from build123d import *

# Parameters (mm, degrees)
CROQUIS2_W              = 50
CROQUIS2_H              = 50
SALIENTE_EXTRUIR1_DEPTH = 1.4
CROQUIS3_R              = 1.6
CORTAR_EXTRUIR1_DEPTH   = 1.4
CROQUIS4_W              = 50
CROQUIS4_H              = 32.2
SALIENTE_EXTRUIR2_DEPTH = 23.2
SALIENTE_EXTRUIR3_DEPTH = 14.6
CROQUIS6_R              = 5
SALIENTE_EXTRUIR4_DEPTH = 16.4


with BuildPart() as part:
    # Croquis2 → Saliente-Extruir1 (new body)
    with BuildSketch(Plane.XY):
        Rectangle(CROQUIS2_W, CROQUIS2_H)
    extrude(amount=SALIENTE_EXTRUIR1_DEPTH)

    # Croquis3 → Cortar-Extruir1 (cut)
    with BuildSketch(Plane.XY.offset(1.4)):
        with Locations((20.4, 22)):
            Circle(CROQUIS3_R)
        with Locations((20.4, -18)):
            Circle(CROQUIS3_R)
        with Locations((-18.1, 22)):
            Circle(CROQUIS3_R)
        with Locations((-18.1, -18)):
            Circle(CROQUIS3_R)
    extrude(amount=-CORTAR_EXTRUIR1_DEPTH, mode=Mode.SUBTRACT)

    # Croquis4 → Saliente-Extruir2 (add)
    with BuildSketch(Plane(origin=(0, 0, 0), x_dir=(-1, 0, 0), z_dir=(0, 0, -1))):
        with Locations((0, 2.75)):
            Rectangle(CROQUIS4_W, CROQUIS4_H)
    extrude(amount=SALIENTE_EXTRUIR2_DEPTH)

    # Croquis5 → Saliente-Extruir3 (add)
    with BuildSketch(Plane.XY.offset(1.4)):
        Polygon((-14.1, -18), (-14.1, -25), (5.9, -25), (5.9, -15), (-14.1, -15), align=None)
    extrude(amount=SALIENTE_EXTRUIR3_DEPTH)

    # Croquis6 → Saliente-Extruir4 (add)
    with BuildSketch(Plane.XY.offset(1.4)):
        with Locations(Location((11.9, -20, 0), (0, 0, 270))):
            Circle(CROQUIS6_R)
    extrude(amount=SALIENTE_EXTRUIR4_DEPTH)


solid = part.part
Check sheet for the modelled part. Datum: model origin and axes. Units: mm. A direction names the side the tool comes from. Round coordinates to 2 decimals unless told otherwise and drop trailing zeros. Loops run counter-clockwise (first coordinate to the right, second up) from the corner with the lowest first, then second, coordinate; pieces in that order, holes last. Notation, with made-up numbers: M -30.75,38.25 L 25.25,38.25 A16 cw 25.25,48.25 Z; hole C 52.25,64 d10. An arc over 180 degrees is marked long. One line per question, with ' | ' between items. Start each with the question number.
Item 1: Section check D-D (x = -2). Record the boundary of the cut face in (y, z).
Item 2: Scan lines: probe 1 along Y at (x, z) = (20.4, 0.6); probe 2 along Y at (x, z) = (5.5, 7.5); probe 3 along Y at (x, z) = (-22, -12.5). Record each from-to range of solid material in increasing order.
Item 3: Section check C-C (z = 12). Record the boundary of the cut face in (x, y), and give its area (3 significant figures).
Item 4: Section check A-A (y = 22). Record the boundary of the cut face in (x, z).
Item 5: Section check B-B (x = -18.1). Record the boundary of the cut face in (y, z).
Item 6: Set-up check for faces 1 (the face through (-4, -20, 16)), 2 (the face through (-4, -15, 9)), 3 (the face through (0, 22, 0)), 4 (the face through (0, -19, 0)): record each of +Z, -Z, +X, -X, +Y, -Y from which the full face is reachable in a straight line by a thin tool's end or side.
Item 7: Gauge pin test, flat ends, axial feed: pin 1 Ø15 at (x, y) = (4, 5.5) entering from +Z; pin 2 Ø5 at (x, y) = (0.5, 20.5) entering from -Z; pin 3 Ø11 at (y, z) = (-18, 11) entering from +X; pin 4 Ø4 at (x, z) = (16, -14) entering from -Y. Record the tip position at first contact, or that the pin passes through.
Item 8: Release check for a two-part mould opening along Y. For faces 5 (the face through (7, -19, 9)), 6 (the face through (22, 22, 1)), 7 (the face through (0, 18.85, -11)) record: released by +Y, released by -Y, zero draft, split by the parting line, or undercut.
Worked out:
1) outline: M -25,0 L -13.35,0 L -13.35,-23.2 L 18.85,-23.2 L 18.85,0 L 25,0 L 25,1.4 L -15,1.4 L -15,16 L -25,16 Z
2) probe 1: -25 to -19.6, -16.4 to 20.4, 23.6 to 25 | probe 2: -25 to -15 | probe 3: -13.35 to 18.85
3) outline: M -14.1,-25 L 5.9,-25 L 5.9,-15 L -14.1,-15 Z; C 11.9,-20 d10 | area: 279 mm^2
4) outline: M -25,0 L -19.7,0 L -19.7,1.4 L -25,1.4 Z; M -16.5,0 L 18.8,0 L 18.8,1.4 L -16.5,1.4 Z; M 22,0 L 25,0 L 25,1.4 L 22,1.4 Z
5) outline: M -25,0 L -19.6,0 L -19.6,1.4 L -25,1.4 Z; M -16.4,0 L -13.35,0 L -13.35,-23.2 L 18.85,-23.2 L 18.85,0 L 20.4,0 L 20.4,1.4 L -16.4,1.4 Z; M 23.6,0 L 25,0 L 25,1.4 L 23.6,1.4 Z
6) face 1: +Z, -X, +Y, -Y | face 2: +Z, +X, -X, +Y | face 3: -Z, +X, -X, +Y | face 4: -Z, +X, -X, -Y
7) pin 1: z = 1.4 | pin 2: z = -23.2 | pin 3: x = 16.9 | pin 4: y = -13.35
8) face 5: split by the parting line | face 6: undercut | face 7: released by +Y
